Check sheet for the modelled part. Datum: model origin and axes. Units: mm. Coordinates: 2 decimals unless noted, no trailing zeros. Write each loop counter-clockwise with the first axis right and the second up, starting at its lowest first coordinate (ties: lowest second). Pieces come first, ordered by that corner, then holes. Notation, with made-up numbers: M 40,-17 L 53,-17 A27 ccw 53,10 Z; hole C 46.5,62.5 d4. An arc over 180 degrees is marked long. Answer as CSV lines item,"result". Start each with the question number.
Q1. Sectioned sample at A-A, the plane y = 0. Record the cut outline in (x, z), then the cut area to 3 significant figures.
Q2. Sectioned sample at C-C, the plane y = -6.5. Record the cut outline in (x, z).
Q3. Sectioned sample at D-D, the plane z = 32. Record the cut outline in (x, y), then the cut area to 3 significant figures.
Q4. Thickness scan on line 1 along Z through (x, y) = (0.65, 0); line 2 along Y through (x, z) = (-0.5, -26); line 3 along Y through (x, z) = (0.6, 23). Record the ranges inside material, lowest first. Write a range as from..to.
Q5. Sectioned sample at B-B, the plane x = 0.2. Record the cut outline in (y, z), then the cut area to 3 significant figures.
Q6. Depth check by flat-ended pin: pin 1 Ø1.5 at (x, y) = (1, -5.5) entering from +Z. Enter the tip coordinate at first touch or a pass-through.
Autodesk Inventor part; units mm, degrees
ref_plane "YZ Plane" through (0, 0, 0) normal (1, 0, 0) x (0, 1, 0)
ref_plane "XZ Plane" through (0, 0, 0) normal (0, 1, 0) x (-1, 0, 0)
ref_plane "XY Plane" through (0, 0, 0) normal (0, 0, 1) x (1, 0, 0)
sketch "Sketch1" plane through (0, 0, 0) normal (1, 0, 0) x (0, 1, 0)
  line L0 (0, -25) -> (0, 25) construction
  line L1 (12.5, -25) -> (12.5, 25)
  line L2 (-12.5, 25) -> (-12.5, -25)
  arc A0 (-12.5, -25) -> (12.5, -25) centre (0, -25) ccw
  arc A1 (12.5, 25) -> (-12.5, 25) centre (0, 25) ccw
  line L3 (23.5288, 0) -> (-21.155, 0)
  circle A2 centre (0, 25) radius 5
  circle A3 centre (0, -25) radius 5
  point P0 (0, 0)
  dimension "d1" = 25
  dimension "d15" = 10
  dimension "d16" = 50
extrude "Extrusion1" add sketch "Sketch1" along normal mid plane 3
properties part number "joint"
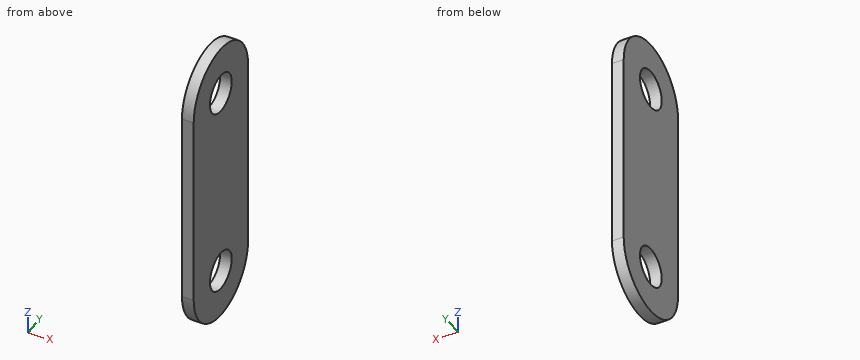
Output:
1,outline,"M -1.5,-37.5 L 1.5,-37.5 L 1.5,-30 L -1.5,-30 Z; M -1.5,-20 L 1.5,-20 L 1.5,20 L -1.5,20 Z; M -1.5,30 L 1.5,30 L 1.5,37.5 L -1.5,37.5 Z"
1,area,"165 mm^2"
2,outline,"M -1.5,-35.68 L 1.5,-35.68 L 1.5,35.68 L -1.5,35.68 Z"
3,outline,"M -1.5,-10.36 L 1.5,-10.36 L 1.5,10.36 L -1.5,10.36 Z"
3,area,"62.1 mm^2"
4,line 1,"z = -37.5..-30, -20..20, 30..37.5"
4,line 2,"y = -12.46..-4.9, 4.9..12.46"
4,line 3,"y = -12.5..-4.58, 4.58..12.5"
5,outline,"M -12.5,-25 A12.5 ccw 12.5,-25 L 12.5,25 A12.5 ccw -12.5,25 Z; hole C 0,-25 d10; hole C 0,25 d10"
5,area,"1,580 mm^2"
6,pin 1,"stops at z = 36.56"
